from build123d import *

# Parameters (mm, degrees)
TORUS_R               = 2
TORUS_ANGLE           = 120
TORUS_PLACEMENT_ANGLE = 204
CYLINDER002_R         = 4
CYLINDER002_DEPTH     = 10
CYLINDER001_R         = 4
CYLINDER001_DEPTH     = 10
CYLINDER_R            = 25
CYLINDER_DEPTH        = 3


with BuildPart() as toro:
    # Torus → Torus (revolve)
    with BuildSketch(Plane.XZ):
        with Locations((11, 0)):
            Circle(TORUS_R)
    revolve(axis=Axis((0, 0, 0), (0, 0, 1)), revolution_arc=TORUS_ANGLE)


with BuildPart() as toro_1:
    # Torus placement: moved
    add(toro.part.moved(Location((0, 0, 2))).rotate(Axis((0, 0, 2), (0, 0, 1)), TORUS_PLACEMENT_ANGLE))


with BuildPart() as cilindro002:
    # Cylinder002 → Cylinder002 (new body)
    with BuildSketch(Plane(origin=(12, 11, -2), x_dir=(1, 0, 0), z_dir=(0, 0, 1))):
        Circle(CYLINDER002_R)
    extrude(amount=CYLINDER002_DEPTH)


with BuildPart() as fusion:
    # Cylinder001 → Cylinder001 (new body)
    with BuildSketch(Plane(origin=(-13, 11, -2), x_dir=(1, 0, 0), z_dir=(0, 0, 1))):
        Circle(CYLINDER001_R)
    extrude(amount=CYLINDER001_DEPTH)

    # Fusion: union Cilindro002
    add(cilindro002.part)


with BuildPart() as cut001:
    # Cylinder → Cylinder (new body)
    with BuildSketch(Plane.XY):
        Circle(CYLINDER_R)
    extrude(amount=CYLINDER_DEPTH)

    # Cut: cut Fusion
    add(fusion.part, mode=Mode.SUBTRACT)

    # Cut001: cut Toro
    add(toro_1.part, mode=Mode.SUBTRACT)


solid = cut001.part
Can you work these out from the model? Positions are in its coordinate system, mm. A direction names the side the tool comes from. Round coordinates to 2 decimals unless told otherwise and drop trailing zeros. Order: outer loops, then holes, each group sorted by start corner. A loop starts at its lowest first (then second) coordinate and runs counter-clockwise, first axis right, second up. Notation, with made-up numbers: M 6.25,86.25 L 33.25,86.25 A30 ccw 33.25,117.25 Z; hole C 24.25,18.5 d3. An arc over 180 degrees is marked long. Use a Markdown table: item, result.
1) If I drill on line 1 along X through (y, z) = (11, 2.1); line 2 along X through (y, z) = (14, 2.3); line 3 along Y through (x, z) = (-13, 1.7), over which ranges is the centre line in solid material (lowest first)?
Geometry says:
| item | result |
|---|---|
| line 1 | x = -22.45 to -17, -9 to 8, 16 to 22.45 |
| line 2 | x = -20.71 to -15.65, -10.35 to 9.35, 14.65 to 20.71 |
| line 3 | y = -21.35 to 7, 15 to 21.35 |
2) Imagine slicing it at C-C (y = 11). List the corners of the cut face in (x, z) for me, then the cut area to 3 significant figures.
Geometry says:
| item | result |
|---|---|
| outline | M -22.45,0 L -17,0 L -17,3 L -22.45,3 Z; M -9,0 L 8,0 L 8,3 L -9,3 Z; M 16,0 L 22.45,0 L 22.45,3 L 16,3 Z |
| area | 86.7 mm² |
3) Imagine slicing it at B-B (z = 1). List the corners of the cut face in (x, y) for me, then the cut area to 3 significant figures.
Geometry says:
| item | result |
|---|---|
| outline | C 0,0 d50; hole C -13,11 d8; hole M -11.63,-5.18 A12.73 ccw 10.3,-7.48 L 7.5,-5.45 A9.27 cw -8.47,-3.77 Z; hole C 12,11 d8 |
| area | 1,780 mm² |
4) I'm going to push flat-ended pins straight in: P1, Ø2, axis at x = -9, y = 17.5, coming from the -Z side; P2, Ø1, axis at x = 16, z = 0.5, coming from the +Y side; P3, Ø7, axis at x = -13, y = 11, coming from the -Z side; P4, Ø1, axis at x = -15.5, z = 2.5, coming from the -Y side. Where does each tip first touch, or does it pass through?
Geometry says:
| item | result |
|---|---|
| P1 | stops at z = 0 |
| P2 | stops at y = 19.62 |
| P3 | passes through |
| P4 | stops at y = -20 |
5) Imagine slicing it at D-D (y = -20). List the corners of the cut face in (x, z) for me, then the cut area to 3 significant figures.
Geometry says:
| item | result |
|---|---|
| outline | M -15,0 L 15,0 L 15,3 L -15,3 Z |
| area | 90.0 mm² |
6) On a 3-axis mill with a long thin cutter (end or side, diameter ignored), from which of +Z, -Z, +X, -X, +Y, -Y can I reach the whole of each face in a straight line? I mean faces 4 (the face through (0, 0, 0)), 5 (the face through (-10.02, -4.46, 1.85)). Say none if no direction works.
Geometry says:
| item | result |
|---|---|
| face 4 | -Z, +X, -X, +Y, -Y |
| face 5 | none |
7) If we mould it in two halves opening along X, with no side actions, what happens to faces 1 (the face through (9.05, 13.7, 1.48)), 2 (the face through (0, 0, 3)), 3 (the face through (23.846, 7.509, 1.479))? For each: +X half, -X half, draft (parallel to the pull), parting line (faces both ways), or undercut.
Geometry says:
| item | result |
|---|---|
| face 1 | undercut |
| face 2 | draft |
| face 3 | parting line |
8) Imagine slicing it at A-A (x = 15). List the corners of the cut face in (y, z) for me, then the cut area to 3 significant figures.
Geometry says:
| item | result |
|---|---|
| outline | M -20,0 L 8.35,0 L 8.35,3 L -20,3 Z; M 13.65,0 L 20,0 L 20,3 L 13.65,3 Z |
| area | 104 mm² |
